from build123d import *

# Parameters (mm, degrees)
SKETCH1_W           = 42
SKETCH1_H           = 42
SKETCH1_R           = 2
SKETCH1_R_2         = 10
BOSS_EXTRUDE1_DEPTH = 7
SKETCH2_R           = 17
SKETCH2_R_2         = 5
BOSS_EXTRUDE2_DEPTH = 15
FILLET1_R           = 5


with BuildPart() as part:
    # Sketch1 → Boss-Extrude1 (new body)
    with BuildSketch(Plane(origin=(0, 0, 0), x_dir=(0, 0, -1), z_dir=(1, 0, 0))):
        Rectangle(SKETCH1_W, SKETCH1_H)
        with Locations((-14.849242405, 14.849242405)):
            Circle(SKETCH1_R, mode=Mode.SUBTRACT)
        with Locations((14.849242405, 14.849242405)):
            Circle(SKETCH1_R, mode=Mode.SUBTRACT)
        with Locations((14.849242405, -14.849242405)):
            Circle(SKETCH1_R, mode=Mode.SUBTRACT)
        with Locations((-14.849242405, -14.849242405)):
            Circle(SKETCH1_R, mode=Mode.SUBTRACT)
        Circle(SKETCH1_R_2, mode=Mode.SUBTRACT)
    extrude(amount=BOSS_EXTRUDE1_DEPTH)

    # Sketch2 → Boss-Extrude2 (add)
    with BuildSketch(Plane(origin=(0, 0, 0), x_dir=(0, 0, -1), z_dir=(1, 0, 0))):
        Circle(SKETCH2_R)
        Circle(SKETCH2_R_2, mode=Mode.SUBTRACT)
    extrude(amount=BOSS_EXTRUDE2_DEPTH)

    # Fillet1
    fillet1_edges = [part.edges().sort_by_distance(p)[0] for p in [
        (3.5, 21, 21),
        (3.5, 21, -21),
        (3.5, -21, -21),
        (3.5, -21, 21),
    ]]
    fillet(fillet1_edges, radius=FILLET1_R)


solid = part.part
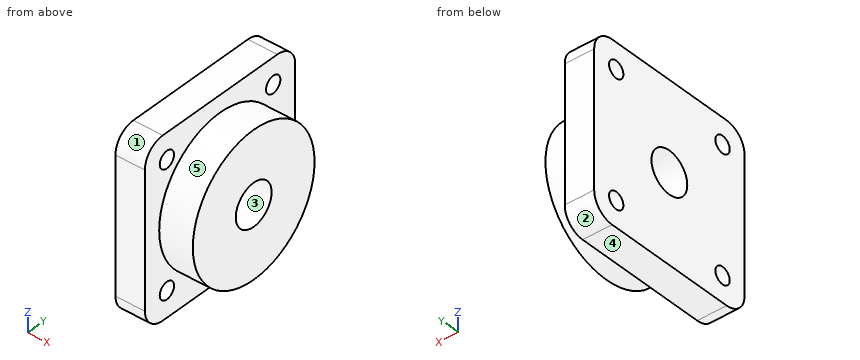
Geometry check sheet. Reference: the model listing, model coordinates, mm. Face numbers are marked on the shaded views. A direction names the side the tool comes from. Round coordinates to 2 decimals unless told otherwise and drop trailing zeros. Order: outer loops, then holes, each group sorted by start corner. A loop starts at its lowest first (then second) coordinate and runs counter-clockwise, first axis right, second up. Notation, with made-up numbers: M -36,25 L -8,25 A11 cw -8,34 Z; hole C 74,-15 d3. An arc over 180 degrees is marked long. Write each question's results on one line, items separated by ' | '. Start each with the question number.
1. Cross-section at A-A on y = 0. Record the boundary of the cut face in (x, z), plus the area to 3 significant figures.
2. Material ranges on L1, parallel to Z at x = 5.25, y = -14; L2, parallel to X at y = 14, z = 17.5; L3, parallel to Z at x = 3.5, y = -16.5, recorded low to high. Write a range as from..to.
3. Cross-section at D-D on x = 10. Record the boundary of the cut face in (y, z), plus the area to 3 significant figures.
4. Set-up check for the marked faces 4 and 5: record each of +Z, -Z, +X, -X, +Y, -Y from which the full face is reachable in a straight line by a thin tool's end or side.
5. Go/stop test with flat-tipped pins: P1, Ø2.5, axis at y = 14.85, z = 14.85, coming from the -X side; P2, Ø1, axis at x = 11.5, y = 15, coming from the -Z side; P3, Ø8, axis at x = 13, z = 10, coming from the +Y side; P4, Ø4, axis at x = 13.5, z = 2, coming from the +Y side. Record where each tip stops, or that it passes through.
6. Cross-section at C-C on y = 14. Record the boundary of the cut face in (x, z).
7. Draft check along Y on the marked faces 1, 2 and 3. Enter one of: pulls with the +Y half, pulls with the -Y half, needs draft (parallel to the pull), parting line crosses it, or undercut.
Resolved:
1) outline: M 0,-21 L 7,-21 L 7,-17 L 15,-17 L 15,-5 L 0,-5 Z; M 0,5 L 15,5 L 15,17 L 7,17 L 7,21 L 0,21 Z | area: 416 mm2
2) L1: -21..-16.66, -13.04..13.04, 16.66..21 | L2: 0..7 | L3: -20.97..-15.98, -13.72..13.72, 15.98..20.97
3) outline: C 0,0 d34; hole C 0,0 d10 | area: 829 mm2
4) face 4: -Z, +X, -X, +Y, -Y | face 5: +X
5) P1: through | P2: z = -8.87 | P3: y = 15.91 | P4: y = 17
6) outline: M 0,-21 L 7,-21 L 7,-16.66 L 0,-16.66 Z; M 0,-13.04 L 7,-13.04 L 7,-9.64 L 15,-9.64 L 15,9.64 L 7,9.64 L 7,13.04 L 0,13.04 Z; M 0,16.66 L 7,16.66 L 7,21 L 0,21 Z
7) face 1: pulls with the -Y half | face 2: pulls with the +Y half | face 3: undercut
